Part print with two shaded views. Sizes in mm from the minimum x, y, z corner. Round coordinates to 2 decimals unless told otherwise and drop trailing zeros. Loops run counter-clockwise (first coordinate to the right, second up) from the corner with the lowest first, then second, coordinate; pieces in that order, holes last.
(1) Cut at B-B on y = 14.25. List the corners of the cut face in (x, z), then the cut area to 3 significant figures.
(2) Cut at C-C on x = 1.15. List the corners of the cut face in (y, z).
(3) Cut at A-A on z = 12.5. List the corners of the cut face in (x, y), then the cut area to 3 significant figures.
(4) Probe probe 1 along Y at (x, z) = (1, 12.5); probe 2 along Y at (x, z) = (1.05, 17); probe 3 along Y at (x, z) = (0.25, 10). List the from-to ranges inside material, lowest first.
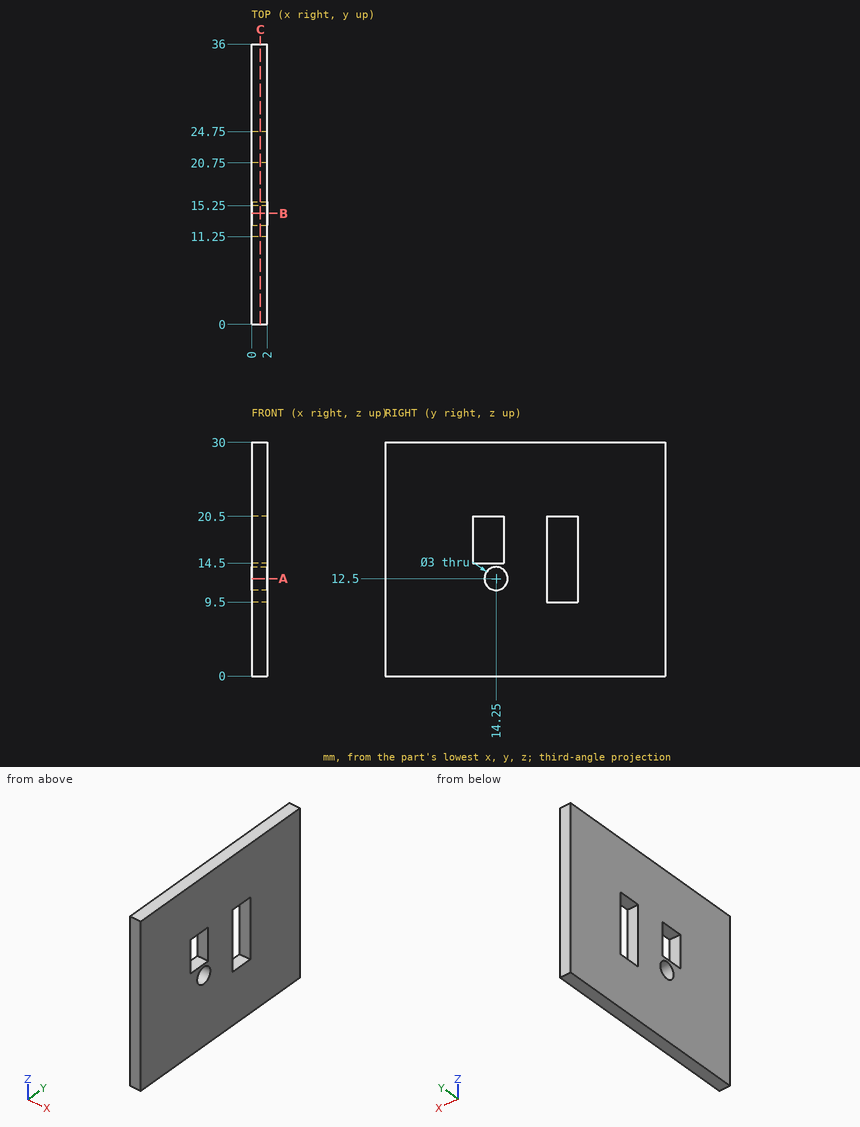
Final values:
1. outline: (0, 0) - (2, 0) - (2, 11) - (0, 11) - close; (0, 14) - (2, 14) - (2, 14.5) - (0, 14.5) - close; (0, 20.5) - (2, 20.5) - (2, 30) - (0, 30) - close
1. area: 42.0 mm2
2. outline: (0, 0) - (36, 0) - (36, 30) - (0, 30) - close; hole (11.25, 14.5) - (15.25, 14.5) - (15.25, 20.5) - (11.25, 20.5) - close; hole circle Ø3 at (14.25, 12.5); hole (20.75, 9.5) - (24.75, 9.5) - (24.75, 20.5) - (20.75, 20.5) - close
3. outline: (0, 0) - (2, 0) - (2, 12.75) - (0, 12.75) - close; (0, 15.75) - (2, 15.75) - (2, 20.75) - (0, 20.75) - close; (0, 24.75) - (2, 24.75) - (2, 36) - (0, 36) - close
3. area: 58.0 mm2
4. probe 1: y = 0 to 12.75, 15.75 to 20.75, 24.75 to 36
4. probe 2: y = 0 to 11.25, 15.25 to 20.75, 24.75 to 36
4. probe 3: y = 0 to 20.75, 24.75 to 36
